```python
from build123d import *

# Parameters (mm, degrees)
SKETCH001_R  = 7.98
PAD001_DEPTH = 60
SKETCH002_R  = 1.85
POCKET_DEPTH = 10
SKETCH_R     = 15.152226
PAD_DEPTH    = 3


with BuildPart() as part:
    # Sketch001 → Pad001 (new body)
    with BuildSketch(Plane.XY.offset(2)):
        Circle(SKETCH001_R)
    extrude(amount=PAD001_DEPTH)

    # Sketch002 → Pocket (cut)
    with BuildSketch(Plane.XY.offset(62)):
        Circle(SKETCH002_R)
    extrude(amount=-POCKET_DEPTH, mode=Mode.SUBTRACT)

    # Sketch → Pad (new body)
    with BuildSketch(Plane(origin=(0, 0, 2), x_dir=(1, 0, 0), z_dir=(0, 0, -1))):
        Circle(SKETCH_R)
    extrude(amount=PAD_DEPTH)


solid = part.part
```
Part model, mm, in its own coordinate system. A direction names the side the tool comes from. Round coordinates to 2 decimals unless told otherwise and drop trailing zeros. Loops run counter-clockwise (first coordinate to the right, second up) from the corner with the lowest first, then second, coordinate; pieces in that order, holes last.
Item 1: Cut at A-A, the plane x = 0. Give the cut face in (y, z), then the cut area to 3 significant figures.
Item 2: Cut at C-C, the plane z = 55.5. Give the cut face in (x, y).
Item 3: Cut at B-B, the plane y = 7. Give the cut face in (x, z).
Item 4: Drill centre lines: line 1 (Y direction, x = 0, z = 55.25); line 2 (Z direction, x = 0, y = 9); line 3 (X direction, y = -0.5, z = 42). Where is each one in solid material? Low to high.
Item 5: Mould opens along X. For faces 3 (the face through (-0.401, -1.806, 57.07)), 4 (the face through (2, -2, 62)), 5 (the face through (0, 0, 52)), 6 (the face through (8.146, -12.776, 0.521)) say: +X half, -X half, draft (parallel to the pull), parting line (faces both ways), or undercut.
Item 6: Drop flat-ended pins along their axis: P1, Ø8, axis at y = -10, z = 27.5, coming from the +X side; P2, Ø1, axis at x = -7.5, y = 7.5, coming from the +Z side; P3, Ø12, axis at y = 10.5, z = 6.5, coming from the +X side. Give the stop position or say it passes through.
Item 7: 3-axis set-ups, long thin cutter, end or side, ignore diameter. For faces 1 (the face through (7, 7, 2)), 2 (the face through (0, 0, -1)): which of +Z, -Z, +X, -X, +Y, -Y reach the whole face in a straight line?
Item 8: Cut at D-D, the plane z = 39. Give the cut face in (x, y).
A:
1. outline: (-15.15, -1) - (15.15, -1) - (15.15, 2) - (7.98, 2) - (7.98, 62) - (1.85, 62) - (1.85, 52) - (-1.85, 52) - (-1.85, 62) - (-7.98, 62) - (-7.98, 2) - (-15.15, 2) - close
1. area: 1,010 mm2
2. outline: circle Ø15.96 at (0, 0); hole circle Ø3.7 at (0, 0)
3. outline: (-13.44, -1) - (13.44, -1) - (13.44, 2) - (3.83, 2) - (3.83, 62) - (-3.83, 62) - (-3.83, 2) - (-13.44, 2) - close
4. line 1: y = -7.98 to -1.85, 1.85 to 7.98
4. line 2: z = -1 to 2
4. line 3: x = -7.96 to 7.96
5. face 3: undercut
5. face 4: draft
5. face 5: undercut
5. face 6: parting line
6. P1: stops at x = 5.26
6. P2: stops at z = 2
6. P3: stops at x = 13.67
7. face 1: +Z
7. face 2: -Z, +X, -X, +Y, -Y
8. outline: circle Ø15.96 at (0, 0)
